Autodesk Inventor part; units mm, degrees
ref_plane "YZ Plane" through (0, 0, 0) normal (1, 0, 0) x (0, 1, 0)
ref_plane "XZ Plane" through (0, 0, 0) normal (0, 1, 0) x (-1, 0, 0)
ref_plane "XY Plane" through (0, 0, 0) normal (0, 0, 1) x (1, 0, 0)
sketch "Sketch2" plane through (0, 0, 0) normal (0, 0, 1) x (1, 0, 0)
  line L0 (-1.7321, 3) -> (1.7321, 3)
  line L1 (1.7321, 3) -> (3.4641, 0)
  line L2 (3.4641, 0) -> (1.7321, -3)
  line L3 (1.7321, -3) -> (-1.7321, -3)
  line L4 (-1.7321, -3) -> (-3.4641, 0)
  line L5 (-3.4641, 0) -> (-1.7321, 3)
  line L6 (-4.8497, 0) -> (4.8497, 0) construction
  circle A0 centre (0, 0) radius 1.5
  dimension "d0" = 6
  dimension "d3" = 3
extrude "Extrusion1" add sketch "Sketch2" along normal blind 15
thread "Thread1"
properties part number "P043_entretoise15par3"
Geometry: final body of the model. Coordinates: model frame, mm. Coordinates: 2 decimals unless noted, no trailing zeros. Write each loop counter-clockwise with the first axis right and the second up, starting at its lowest first coordinate (ties: lowest second). Pieces come first, ordered by that corner, then holes. Notation, with made-up numbers: M -24,-38 L 24,-38 A25 ccw 24,-12 Z; hole C 6.5,-8.75 d9. An arc over 180 degrees is marked long. Answer as CSV lines item,"result". Start each with the question number.
Q1. Cut plane A-A on x = 0. Return the cut outline in (y, z).
Q2. Line query: line 1 (Y direction, x = 0, z = 8); line 2 (X direction, y = -0.05, z = 4.5); line 3 (X direction, y = -0.5, z = 6). Output: solid intervals per line, ascending. Write a range as from..to.
Q3. Mould query, pull axis Y, two halves, no side actions, for faces 1 (the flat face through (-2.6, -1.5, 7.4)), 2 (the flat face through (0, 3, 7)), 3 (the cylindrical face through (-1.5, -0.07, 7.4)), 4 (the flat face through (1.5, 0.7, 0)). Classes: released by +Y, released by -Y, zero draft, split by the parting line, or undercut.
Q4. Cut plane B-B on y = 0.75. Return the cut outline in (x, z), then the cut area to 3 significant figures.
Q5. Cut plane D-D on y = 2.6. Return the cut outline in (x, z), then the cut area to 3 significant figures.
Q6. Cut plane C-C on z = 8.5. Return the cut outline in (x, y).
Q7. Pin query (flat end, axial travel): P1, Ø2, axis at y = 0.5, z = 6.5, coming from the +X side. Return the tip coordinate at first contact, or that it passes through.
Findings below:
1,outline,"M -3,0 L -1.5,0 L -1.5,15 L -3,15 Z; M 1.5,0 L 3,0 L 3,15 L 1.5,15 Z"
2,line 1,"y = -3..-1.5, 1.5..3"
2,line 2,"x = -3.44..-1.5, 1.5..3.44"
2,line 3,"x = -3.18..-1.41, 1.41..3.18"
3,face 1,"released by -Y"
3,face 2,"released by +Y"
3,face 3,"undercut"
3,face 4,"zero draft"
4,outline,"M -3.03,0 L -1.3,0 L -1.3,15 L -3.03,15 Z; M 1.3,0 L 3.03,0 L 3.03,15 L 1.3,15 Z"
4,area,"52.0 mm2"
5,outline,"M -1.96,0 L 1.96,0 L 1.96,15 L -1.96,15 Z"
5,area,"58.9 mm2"
6,outline,"M -3.46,0 L -1.73,-3 L 1.73,-3 L 3.46,0 L 1.73,3 L -1.73,3 Z; hole C 0,0 d3"
7,P1,"stops at x = 3.46"
